The listing builds one solid part. Answer for the finished solid, in the listing's coordinates (mm). A direction names the side the tool comes from. Give positions to 0.01 mm unless a question says otherwise; leave off trailing zeros. Order: outer loops, then holes, each group sorted by start corner. A loop starts at its lowest first (then second) coordinate and runs counter-clockwise, first axis right, second up. Notation, with made-up numbers: M -1.75,53.5 L 53.25,53.5 A34 cw 53.25,89.5 Z; hole C -16.75,30.25 d3. An arc over 180 degrees is marked long. Answer as a JSON object with one key per item and string values. Group by question number.
Autodesk Inventor part; units mm, degrees
ref_plane "Plano de trabalho1" through (111, 0, 0) normal (1, 0, 0) x (0, 0, -1)
ref_plane "YZ Plane" through (0, 0, 0) normal (1, 0, 0) x (0, 1, 0)
ref_plane "XZ Plane" through (0, 0, 0) normal (0, 1, 0) x (-1, 0, 0)
sketch "Esboço1" plane through (0, 0, 0) normal (1, 0, 0) x (0, 1, 0)
  line L0 (0, 0) -> (45, 0)
  line L1 (45, 0) -> (45, -69)
  line L2 (45, -69) -> (0, -69)
  line L3 (0, -69) -> (0, 0)
  dimension "d0" = 45
  dimension "d1" = 69
extrude "Extrusão1" add sketch "Esboço1" along normal blind 10
sketch "Esboço2" plane through (10, 0, 0) normal (1, 0, 0) x (0, 0, -1)
  line L0 (0, 45) -> (0, 0)
  point P0 (22, 29.1579)
  dimension "d4" = 22
hole "Furo1" at (10, 29.1579, -22) direction (-1, 0, 0) diameter 16 end through all
ref_plane "Plano de trabalho1" through (111, 0, 0) normal (1, 0, 0) x (0, 0, -1)
sketch "Esboço3" plane through (111, 0, 0) normal (1, 0, 0) x (0, 0, -1)
  circle A0 centre (50, -30) radius 19
  line L0 (69, 0) -> (69, 45)
  line L1 (69, 45) -> (0, 45)
  point P0 (0, 0)
  dimension "d13" = 38
  dimension "d14" = 75
extrude "Extrusão2" add sketch "Esboço3" against normal blind 25
sketch "Esboço4" plane through (0, 0, -69) normal (0, 0, -1) x (-1, 0, 0)
  line L0 (-10, 0) -> (-84, 0)
  line L1 (-89, -5) -> (-89, -30)
  line L2 (-89, -30) -> (-99, -30)
  line L3 (-99, -30) -> (-99, -5)
  line L4 (-84, 10) -> (-10, 10)
  line L5 (-10, 10) -> (-10, 0)
  line L6 (-111, -11) -> (-111, -49) construction
  line L7 (-111, -30) -> (-86, -30) construction
  line L8 (-86, -49) -> (-86, -11) construction
  arc A0 (-84, 0) -> (-89, -5) centre (-84, -5) ccw
  arc A1 (-84, 10) -> (-99, -5) centre (-84, -5) ccw
  point P0 (0, 0)
  dimension "d17" = 3
  dimension "d18" = 10
  dimension "d19" = 10
  dimension "d20" = 5
  dimension "d21" = 15
extrude "Extrusão3" add sketch "Esboço4" against normal blind 38
sketch "Esboço5" plane through (10, 0, 0) normal (1, 0, 0) x (0, 0, -1)
  line L0 (69, 10) -> (31, 10)
  line L1 (45, 10) -> (55, 10)
  line L2 (55, 10) -> (55, 20)
  line L3 (55, 20) -> (45, 20)
  line L4 (45, 20) -> (45, 10)
  line L5 (31, 10) -> (31, -5)
  point P0 (0, 0)
  dimension "d24" = 10
  dimension "d25" = 10
  dimension "d26" = 14
sketch3d "Esboço 3D1"
  line L0 (10, 10, -69) -> (84, 10, -69)
  arc A0 (84, 10, -69) -> (99, -5, -69) centre (84, -5, -69) ccw
  line L1 (99, -5, -69) -> (99, -30, -69)
sweep "Varredura1" add profiles "Esboço5" path "Esboço 3D1"
fillet "Arredondamento1" radius 25 1 edges at (10, 20, -50)
fillet "Arredondamento2" radius 30 1 edges at (10, 5, -31)
sketch "Esboço6" plane through (111, -30, -50) normal (1, 0, 0) x (0, 0, -1)
  circle A0 centre (0, 0) radius 19
  point P0 (-50, 30)
hole "Furo2" at (111, -30, -50) direction (-1, 0, 0) diameter 16 end through all
properties part number "Peça teste 5" material "Prata"
Item 1: Flat-ended cylindrical pins translate along their axes: P1, Ø7, axis at x = 64.5, z = -62, coming from the +Y side; P2, Ø6, axis at x = 97.5, y = -38, coming from the -Z side; P3, Ø3, axis at x = 54.5, z = -48, coming from the +Y side. Find the tip coordinate at first contact, or state that the pin passes through.
Item 2: A tool of negligible diameter and unlimited length cuts with its end or side. For faces 5 (the flat face through (48, 10, -38)), 6 (the flat face through (63, 12, -55)), 7 (the flat face through (76, 4, -31)), from which of +Z, -Z, +X, -X, +Y, -Y can it reach the whole face along a straight path? Write none if from no direction.
Item 3: Consider probe 1 along Z at (x, y) = (101.75, -30); probe 2 along Y at (x, z) = (104, -50); probe 3 along Y at (x, z) = (2, -22). Determine where each line is inside the solid, lowest interval first. Write a range as from..to.
Item 4: Section C-C (x = 71.5) is taken. Determine the outline of the cut face in (y, z), and give its area (3 significant figures).
Item 5: Section D-D (y = 11.5) is taken. Determine the outline of the cut face in (x, z).
Item 6: Section B-B (y = -35.5) is taken. Determine the outline of the cut face in (x, z).
Item 7: Determine the mould class of faces 1 (the cylindrical face through (87, -1, -50)), 2 (the cylindrical face through (4.93, 34.026, -15.651)), 3 (the cylindrical face through (18.555, 4.93, -21.979)), 4 (the flat face through (60, 20, -50)) for opening direction Y: released by +Y, released by -Y, zero draft, split by the parting line, or undercut.
Values found:
{
 "1": {"P1": "stops at y = 10", "P2": "stops at z = -68.33", "P3": "stops at y = 20"},
 "2": {"face 5": "+Z, +X, +Y", "face 6": "-Z, +X, +Y", "face 7": "+Z, +X, +Y, -Y"},
 "3": {"probe 1": "z = -69..-58, -42..-31", "probe 2": "y = -49..-38, -22..10", "probe 3": "y = 0..21.16, 37.16..45"},
 "4": {"outline": "M 0,-69 L 10,-69 L 10,-55 L 20,-55 L 20,-45 L 10,-45 L 10,-31 L 0,-31 Z", "area": "480 mm^2"},
 "5": {"outline": "M 0,-69 L 10,-69 L 10,-55 L 102.78,-55 L 102.78,-45 L 10,-45 L 10,0 L 0,0 Z"},
 "6": {"outline": "M 86,-68.19 L 111,-68.19 L 111,-55.81 L 86,-55.81 Z; M 86,-44.19 L 111,-44.19 L 111,-31.81 L 86,-31.81 Z"},
 "7": {"face 1": "undercut", "face 2": "undercut", "face 3": "zero draft", "face 4": "released by +Y"}
}
